The listing builds one solid part. Answer for the finished solid, in the listing's coordinates (mm). Face numbers are marked on the shaded views. Round coordinates to 2 decimals unless told otherwise and drop trailing zeros. Loops run counter-clockwise (first coordinate to the right, second up) from the corner with the lowest first, then second, coordinate; pieces in that order, holes last. Notation, with made-up numbers: (-16.75, 28.25) - (30.25, 28.25) arc R21 ccw to (30.25, 37.25) - close; hole circle Ø5 at (-33, 19.5). An arc over 180 degrees is marked (long way). One line per question, with ' | ' between items. Start each with the question number.
from build123d import *

# Parameters (mm, degrees)
SKETCH1_W                = 76.2
SKETCH1_H                = 17.78
BOSS_EXTRUDE1_DEPTH      = 7.62
FILLET1_R                = 8.89
CUT_EXTRUDE8_DEPTH       = 40.858581259
CUT_EXTRUDE9_DEPTH       = 40.858581259
CUT_EXTRUDE10_DEPTH      = 40.858581259
FILLET5_R                = 8.89
FILLET6_R                = 1.27
CUT_EXTRUDE11_DEPTH      = 40.858581259
SKETCH11_R               = 0.508
CUT_EXTRUDE12_DEPTH      = 40.858581259
CUT_EXTRUDE14_DEPTH      = 40.858581259
CUT_EXTRUDE14_DEPTH_BACK = 40.858581259
FILLET7_R                = 20.32


# Some blends are built 0.0001 mm under size
with BuildPart() as part:
    # Sketch1 → Boss-Extrude1 (new body)
    with BuildSketch(Plane(origin=(0, 0, 0), x_dir=(1, 0, 0), z_dir=(0, 1, 0))):
        Rectangle(SKETCH1_W, SKETCH1_H)
    extrude(amount=BOSS_EXTRUDE1_DEPTH)

    # Fillet1
    fillet1_edges = [part.edges().sort_by_distance(p)[0] for p in [
        (-38.1, 3.81, -8.89),
        (-38.1, 3.81, 8.89),
    ]]
    fillet(fillet1_edges, radius=FILLET1_R - 0.0001)  # a hair under: the kernel refuses the full size

    # Sketch2 → Cut-Extrude8 (cut, through all)
    with BuildSketch(Plane(origin=(0, 7.62, 0), x_dir=(1, 0, 0), z_dir=(0, 1, 0))):
        with BuildLine():
            Line((38.1, -3.81), (38.1, 3.81))
            Line((38.1, 3.81), (32.835440572, 3.81))
            Line((32.835440572, 3.81), (32.835440572, 4.572))
            Line((32.835440572, 4.572), (-27.94, 5.588))
            ThreePointArc((-27.94, 5.588), (-33.528, 0), (-27.94, -5.588))
            Line((-27.94, -5.588), (32.835440572, -4.572))
            Line((32.835440572, -4.572), (32.835440572, -3.81))
            Line((32.835440572, -3.81), (38.1, -3.81))
        make_face()
    extrude(amount=-CUT_EXTRUDE8_DEPTH, mode=Mode.SUBTRACT)

    # Sketch8 → Cut-Extrude9 (cut, through all)
    with BuildSketch(Plane(origin=(0, 7.62, 0), x_dir=(1, 0, 0), z_dir=(0, 1, 0))):
        Polygon((-29.21, 8.89), (38.1, 6.35), (38.1, 8.89), align=None)
    cut_extrude9 = extrude(amount=-CUT_EXTRUDE9_DEPTH, mode=Mode.SUBTRACT)

    # Mirror5: Cut-Extrude9 across plane
    add(cut_extrude9.mirror(Plane.XY), mode=Mode.SUBTRACT)

    # Sketch9 → Cut-Extrude10 (cut, through all)
    with BuildSketch(Plane(origin=(0, 7.62, 0), x_dir=(1, 0, 0), z_dir=(0, 1, 0))):
        Polygon((16.543360441, 7.163458097), (38.1, 5.185109732), (38.1, 6.35), align=None)
    cut_extrude10 = extrude(amount=-CUT_EXTRUDE10_DEPTH, mode=Mode.SUBTRACT)

    # Mirror6: Cut-Extrude10 across plane
    add(cut_extrude10.mirror(Plane.XY), mode=Mode.SUBTRACT)

    # Fillet5
    # the kernel refuses this fillet: 8.89 mm, written as the material it adds along each edge
    with BuildSketch(Plane(origin=(32.835440572, 7.62, 4.572), x_dir=(-0.999860295571869, 0, 0.01671494358156383), z_dir=(0, -1, 0))) as fillet5_piece_1:
        with BuildLine():
            CenterArc((3.588094431, 8.89), FILLET5_R, 246.106185647, 23.893814353)
            Line((-0.012736787, 0.761893545), (-0.084753411, 0.599331416))
            ThreePointArc((-0.084753411, 0.599331416), (-0.184143554, 0.377974856), (-0.177775161, -0.002971917))
            Line((-0.177775161, -0.002971917), (0, -0.1778))
            Line((0, -0.1778), (3.588094431, -0.1778))
            Line((3.588094431, -0.1778), (3.588094431, 0))
        make_face()
    extrude(amount=7.62)
    with BuildSketch(Plane(origin=(32.835440572, 7.62, -4.572), x_dir=(0, 0, 1), z_dir=(0, -1, 0))) as fillet5_piece_2:
        with BuildLine():
            CenterArc((8.828783232, 3.736189007), FILLET5_R, 180.957740323, 23.893814353)
            Line((-0.059974796, 3.587593158), (-0.237749957, 3.584621241))
            Line((-0.237749957, 3.584621241), (-0.177775161, -0.002971917))
            Line((-0.177775161, -0.002971917), (0, -0.1778))
            ThreePointArc((0, -0.1778), (0.381, -0.1778), (0.600664335, -0.07472378))
            Line((0.600664335, -0.07472378), (0.762, 0))
        make_face()
    extrude(amount=7.62)

    # Fillet6
    fillet6_edges = [part.edges().sort_by_distance(p)[0] for p in [
        (38.1, 3.81, -5.185109732),
        (38.1, 3.81, 5.185109732),
    ]]
    fillet(fillet6_edges, radius=FILLET6_R)

    # Sketch10 → Cut-Extrude11 (cut, through all)
    with BuildSketch(Plane(origin=(0, 7.62, 0), x_dir=(1, 0, 0), z_dir=(0, 1, 0))):
        Polygon((32.835440572, 3.81), (38.086687384, 4.209729588), (38.737760676, 3.81), align=None)
    cut_extrude11 = extrude(amount=-CUT_EXTRUDE11_DEPTH, mode=Mode.SUBTRACT)

    # Mirror7: Cut-Extrude11 across plane
    add(cut_extrude11.mirror(Plane.XY), mode=Mode.SUBTRACT)

    # Sketch11 → Cut-Extrude12 (cut, through all)
    with BuildSketch(Plane(origin=(0, 7.62, 0), x_dir=(1, 0, 0), z_dir=(0, 1, 0))):
        with Locations((37.070687384, 4.132390762)):
            Circle(SKETCH11_R)
    cut_extrude12 = extrude(amount=-CUT_EXTRUDE12_DEPTH, mode=Mode.SUBTRACT)

    # Mirror8: Cut-Extrude12 across plane
    add(cut_extrude12.mirror(Plane.XY), mode=Mode.SUBTRACT)

    # Sketch13 → Cut-Extrude14 (cut, two sides: drawn at the far end of the back side and taken through both)
    with BuildSketch(Plane.XY.offset(-CUT_EXTRUDE14_DEPTH_BACK)):
        Polygon((-6.333319779, 7.62), (16.543360441, 5.594868468), (38.086687384, 3.194451795), (38.086687384, 7.62), align=None)
    extrude(amount=CUT_EXTRUDE14_DEPTH + CUT_EXTRUDE14_DEPTH_BACK, mode=Mode.SUBTRACT)

    # Fillet7
    fillet7_edges = [part.edges().sort_by_distance(p)[0] for p in [
        (32.835440572, 1.889780071, -3.81),
        (32.835440572, 1.889780071, 3.81),
    ]]
    fillet(fillet7_edges, radius=FILLET7_R)


solid = part.part
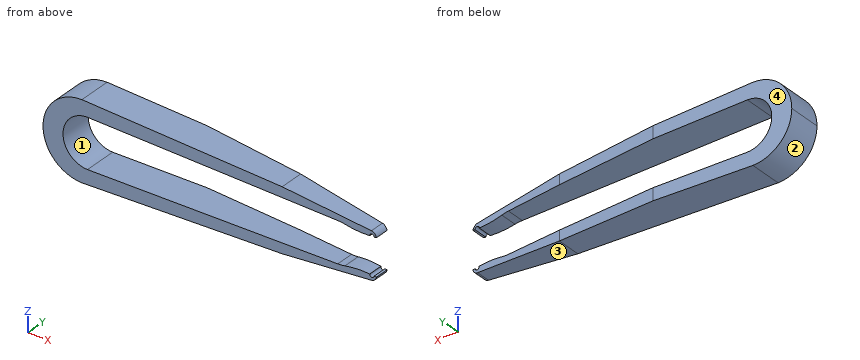
(1) Determine the mould class of the marked faces 1, 2, 3 and 4 for opening direction X: pulls with the +X half, pulls with the -X half, needs draft (parallel to the pull), parting line crosses it, or undercut.
(2) Find section D-D on z = -1.75. Write down the section's boundary in (x, y).
(3) Each of these flat-tipped pins is pushed along its axis until it touches: P1, Ø1.5, axis at y = 2, z = -5, coming from the -X side; P2, Ø4, axis at x = -11, y = 4.5, coming from the +Z side; P3, Ø2, axis at x = 8.5, z = -6, coming from the -Y side; P4, Ø2, axis at y = 4.5, z = 2.5, coming from the +X side. Where does it stop, or does it pass through?
(4) Consider L1, parallel to Z at x = -11.5, y = 1.25; L2, parallel to Z at x = 15.5, y = 0.75; L3, parallel to X at y = 4.25, z = 0.25. Determine where each line is inside the solid, lowest interval first.
(5) Find section A-A on x = -11. Write down the section's boundary in (y, z).
(6) Find section C-C on x = 7. Write down the section's boundary in (y, z).
Answer below:
1) face 1: undercut | face 2: pulls with the -X half | face 3: pulls with the +X half | face 4: needs draft
2) outline: (-37.93, 0) - (-33.25, 0) - (-33.25, 7.62) - (-37.93, 7.62) - close
3) P1: x = -37.02 | P2: z = 8.28 | P3: y = 0 | P4: x = -32.3
4) L1: -8.22 to -5.31, 5.31 to 8.22 | L2: -7.2 to -4.86, 4.86 to 7.2 | L3: -38.1 to -33.52
5) outline: (0, -8.2) - (7.62, -8.2) - (7.62, -5.3) - (0, -5.3) - close; (0, 5.3) - (7.62, 5.3) - (7.62, 8.2) - (0, 8.2) - close
6) outline: (0, -7.52) - (6.44, -7.52) - (6.44, -5) - (0, -5) - close; (0, 5) - (6.44, 5) - (6.44, 7.52) - (0, 7.52) - close
